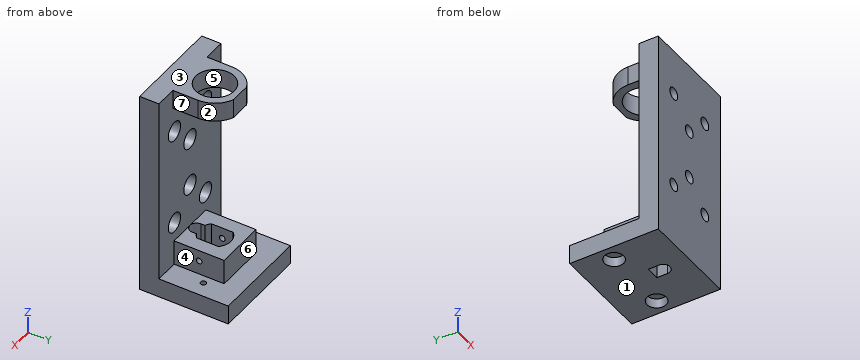
Autodesk Inventor part; units mm, degrees
ref_plane "Work Plane1" through (0, 0, 58.4) normal (0, 0, 1) x (1, 0, 0)
ref_plane "YZ Plane" through (0, 0, 0) normal (1, 0, 0) x (0, 1, 0)
ref_plane "XZ Plane" through (0, 0, 0) normal (0, 1, 0) x (-1, 0, 0)
sketch "Sketch1" plane through (0, 0, 0) normal (0, 0, 1) x (1, 0, 0)
  line L0 (-22.1831, 0) -> (-47.5831, 0)
  line L1 (0, 0) -> (50.8, 0)
  line L2 (50.8, 0) -> (50.8, 5)
  line L3 (50.8, 5) -> (50.8, 10)
  line L4 (50.8, 10) -> (50.8, 36)
  line L5 (50.8, 36) -> (50.8, 46)
  line L6 (50.8, 46) -> (0, 46)
  line L7 (0, 46) -> (0, 0)
  dimension "d0" = 25.4
  dimension "d1" = 50.8
  dimension "d2" = 5
  dimension "d3" = 5
  dimension "d4" = 26
  dimension "d5" = 10
extrude "Extrusion1" add sketch "Sketch1" along normal blind 10
sketch "Sketch2" plane through (0, 0, 10) normal (0, 0, 1) x (1, 0, 0)
  line L0 (50.8, 0) -> (50.8, 46)
  line L1 (50.8, 46) -> (0, 46)
  line L2 (0, 46) -> (0, 0)
  line L3 (0, 0) -> (50.8, 0)
  line L4 (0, 46) -> (0, 0)
  line L5 (0, 0) -> (50.8, 0)
  line L6 (50.8, 0) -> (50.8, 46)
  line L7 (50.8, 0) -> (50.8, 10)
  line L8 (50.8, 10) -> (0, 10)
  line L9 (0, 0) -> (0, 10)
  dimension "d8" = 10
extrude "Extrusion2" add sketch "Sketch2" along normal blind 87.5 contours L3 L2 L8 L0
sketch "Sketch3" plane through (0, 0, 10) normal (0, 0, 1) x (1, 0, 0)
  line L0 (0, 10) -> (50.8, 10)
  line L1 (50.8, 10) -> (50.8, 46)
  line L2 (50.8, 46) -> (0, 46)
  line L3 (0, 46) -> (0, 10)
  line L4 (12.4, 36) -> (38.4, 36)
  line L5 (38.4, 36) -> (38.4, 10)
  line L6 (38.4, 10) -> (12.4, 10)
  line L7 (12.4, 10) -> (12.4, 36)
  line L8 (17.4, 31) -> (33.4, 31)
  line L9 (33.4, 31) -> (33.4, 15)
  line L10 (33.4, 15) -> (17.4, 15)
  line L11 (17.4, 15) -> (17.4, 31)
  point P0 (0, 0)
  dimension "d1" = 50.8
  dimension "d12" = 38.4
  dimension "d13" = 10
  dimension "d14" = 5
  dimension "d15" = 5
  dimension "d16" = 16
  dimension "d17" = 16
  dimension "d18" = 5
  dimension "d19" = 5
  dimension "d24" = 26
  dimension "d26" = 26
extrude "Extrusion3" add sketch "Sketch3" along normal blind 13 contours L7 L4 L5 L0 | L8 L9 L10 L11
sketch "Sketch5" plane through (0, 0, 0) normal (0, 0, -1) x (-1, 0, 0)
  line L0 (-12.4, 36) -> (-38.4, 36)
  line L1 (-38.4, 36) -> (-38.4, 10)
  line L2 (-12.4, 10) -> (-12.4, 36)
  line L3 (0, 10) -> (-12.4, 10)
  line L4 (-50.8, 10) -> (-50.8, 46)
  line L5 (-50.8, 46) -> (0, 46)
  line L6 (0, 46) -> (0, 10)
  line L7 (0, 0) -> (-50.8, 0)
  line L8 (-50.8, 0) -> (-50.8, 10)
  line L9 (-50.8, 10) -> (0, 10)
  line L10 (0, 10) -> (0, 0)
  circle A0 centre (-42.8, 28) radius 1.42
  circle A1 centre (-8, 28) radius 1.42
  line L11 (-38.4, 10) -> (-50.8, 10)
  dimension "d29" = 2.84
  dimension "d30" = 2.84
  dimension "d31" = 8
  dimension "d32" = 8
  dimension "d33" = 8
  dimension "d34" = 8
extrude "Extrusion5" cut sketch "Sketch5" against normal blind 26 contours A0 | A1
sketch "Sketch9" plane through (0, 0, 0) normal (0, 0, -1) x (-1, 0, 0)
  circle A0 centre (-8, 28) radius 1.42
  circle A1 centre (-42.8, 28) radius 1.42
  line L0 (-50.8, 0) -> (-50.8, 46)
  line L1 (0, 0) -> (-50.8, 0)
  line L2 (0, 46) -> (0, 0)
  line L3 (-50.8, 46) -> (0, 46)
  circle A2 centre (-42.8, 28) radius 1.42
  circle A3 centre (-42.8, 28) radius 5
  circle A4 centre (-8, 28) radius 1.42
  circle A5 centre (-8, 28) radius 5
  dimension "d55" = 10
  dimension "d56" = 10
extrude "Extrusion9" cut sketch "Sketch9" against normal blind 5 contours A3 | A5
sketch "Sketch7" plane through (0, 0, 23) normal (0, 0, 1) x (1, 0, 0)
  line L0 (12.4, 36) -> (12.4, 10)
  line L1 (38.4, 10) -> (38.4, 36)
  line L2 (38.4, 36) -> (12.4, 36)
  circle A0 centre (25.4, 23) radius 8.25
  circle A1 centre (25.4, 23) radius 6
  line L3 (19.4, 28.6624) -> (19.4, 17.3376)
  line L4 (38.4, 10) -> (12.4, 10)
  line L5 (31.4, 28.6624) -> (31.4, 17.3376)
  point P0 (0, 0)
  dimension "d42" = 26
  dimension "d43" = 16.5
  dimension "d45" = 13
  dimension "d46" = 12
  dimension "d59" = 26
  dimension "d61" = 0
  dimension "d62" = 180
  dimension "d69" = 0
  dimension "d99" = 13
extrude "Extrusion7" cut sketch "Sketch7" against normal blind 14 contours L5 A1 L3 A0 | A0 L3 A1 L5 | A1
sketch "Sketch10" plane through (38.4, 10, 10) normal (1, 0, 0) x (0, 0, -1)
  line L0 (-13, 7.3376) -> (-13, 18.6624)
  line L1 (-13, 7.3376) -> (1, 7.3376)
  line L2 (1, 7.3376) -> (1, 18.6624)
  line L3 (-13, 18.6624) -> (1, 18.6624)
  circle A0 centre (-7.25, 13) radius 1.5
  point P0 (10, -10)
  dimension "d63" = 3
  dimension "d64" = 8.25
  dimension "d65" = 11.3247
  dimension "d66" = 5.6624
extrude "Extrusion10" cut sketch "Sketch10" against normal through all contours A0
sketch "Sketch11" plane through (0, 10, 97.5) normal (0, 1, 0) x (1, 0, 0)
  line L0 (38.4, 87.5) -> (38.4, 74.5)
  line L1 (38.4, 74.5) -> (12.4, 74.5)
  line L2 (12.4, 74.5) -> (12.4, 87.5)
  line L3 (0, 87.5) -> (12.4, 87.5)
  line L4 (0, 87.5) -> (0, 0)
  line L5 (50.8, 0) -> (0, 0)
  line L6 (50.8, 87.5) -> (50.8, 0)
  line L7 (38.4, 87.5) -> (50.8, 87.5)
  circle A0 centre (50.8, 77.2) radius 3.175
  circle A1 centre (38.1, 64.5) radius 3.175
  line L8 (38.4, 74.5) -> (12.4, 74.5)
  line L9 (38.4, 74.5) -> (25.4, 74.5)
  circle A2 centre (25.4, 77.2) radius 3.175
  circle A3 centre (12.7, 64.5) radius 3.175
  circle A4 centre (0, 77.2) radius 3.175
  circle A5 centre (-12.7, 64.5) radius 3.175
  circle A6 centre (-25.4, 77.2) radius 3.175
  circle A7 centre (-38.1, 64.5) radius 3.175
  circle A8 centre (50.8, 51.8) radius 3.175
  circle A9 centre (38.1, 39.1) radius 3.175
  circle A10 centre (25.4, 51.8) radius 3.175
  circle A11 centre (12.7, 39.1) radius 3.175
  circle A12 centre (0, 51.8) radius 3.175
  circle A13 centre (-12.7, 39.1) radius 3.175
  circle A14 centre (-25.4, 51.8) radius 3.175
  circle A15 centre (-38.1, 39.1) radius 3.175
  circle A16 centre (50.8, 26.4) radius 3.175
  circle A17 centre (38.1, 13.7) radius 3.175
  circle A18 centre (25.4, 26.4) radius 3.175
  circle A19 centre (12.7, 13.7) radius 3.175
  circle A20 centre (0, 26.4) radius 3.175
  circle A21 centre (-12.7, 13.7) radius 3.175
  circle A22 centre (-25.4, 26.4) radius 3.175
  circle A23 centre (-38.1, 13.7) radius 3.175
  circle A24 centre (50.8, 1) radius 3.175
  circle A25 centre (38.1, -11.7) radius 3.175
  circle A26 centre (25.4, 1) radius 3.175
  circle A27 centre (12.7, -11.7) radius 3.175
  circle A28 centre (0, 1) radius 3.175
  circle A29 centre (-12.7, -11.7) radius 3.175
  circle A30 centre (-25.4, 1) radius 3.175
  circle A31 centre (-38.1, -11.7) radius 3.175
  point P0 (0, 97.5)
  dimension "d70" = 26
  dimension "d71" = 6.35
  dimension "d72" = 6.35
  dimension "d73" = 13
  dimension "d75" = 12.7
  dimension "d76" = 12.7
  dimension "d77" = 10.3
  dimension "d78" = 13
  dimension "d82" = 25.4
  dimension "d85" = 25.4
  dimension "d88" = 12.7
extrude "Extrusion11" cut sketch "Sketch11" against normal blind 10 contours A1 | A3 | A10
sketch "Sketch12" plane through (0, 10, 97.5) normal (0, 1, 0) x (1, 0, 0)
  circle A0 centre (38.1, 64.5) radius 3.175
  circle A1 centre (25.4, 51.8) radius 3.175
  circle A2 centre (12.7, 64.5) radius 3.175
  line L0 (38.4, 87.5) -> (38.4, 74.5)
  line L1 (38.4, 74.5) -> (12.4, 74.5)
  line L2 (12.4, 74.5) -> (12.4, 87.5)
  line L3 (0, 87.5) -> (12.4, 87.5)
  line L4 (0, 87.5) -> (0, 0)
  line L5 (50.8, 0) -> (0, 0)
  line L6 (50.8, 87.5) -> (50.8, 0)
  line L7 (38.4, 87.5) -> (50.8, 87.5)
  circle A3 centre (12.7, 64.5) radius 5
  circle A4 centre (25.4, 51.8) radius 5
  circle A5 centre (38.1, 64.5) radius 3.175
  circle A6 centre (38.1, 64.5) radius 5
  point P0 (0, 97.5)
  dimension "d91" = 10
  dimension "d92" = 10
  dimension "d93" = 10
extrude "Extrusion12" cut sketch "Sketch12" against normal blind 5 contours A0 | A1 | A2 | A3 | A4 | A6
sketch "Sketch14" plane through (0, 0, 97.5) normal (0, 0, 1) x (1, 0, 0)
  line L0 (7.7, 5) -> (17.7, 5)
  line L1 (50.8, 10) -> (0, 10)
  line L2 (0, 10) -> (0, 0)
  line L3 (0, 0) -> (50.8, 0)
  line L4 (50.8, 0) -> (50.8, 10)
  circle A0 centre (25.4, 23) radius 10
  circle A1 centre (25.4, 23) radius 14
  line L5 (0, 46) -> (0, 0)
  line L6 (0, 0) -> (50.8, 0)
  line L7 (50.8, 0) -> (50.8, 10)
  line L8 (50.8, 10) -> (0, 10)
  line L9 (0, 10) -> (0, 0)
  circle A2 centre (8, 28) radius 1.42
  circle A3 centre (42.8, 28) radius 1.42
  line L10 (38.4, 36) -> (38.4, 10)
  line L11 (38.4, 10) -> (50.8, 10)
  line L12 (50.8, 10) -> (50.8, 46)
  line L13 (50.8, 46) -> (0, 46)
  line L14 (0, 46) -> (0, 10)
  line L15 (0, 10) -> (12.4, 10)
  line L16 (12.4, 10) -> (12.4, 36)
  line L17 (12.4, 36) -> (38.4, 36)
  circle A4 centre (8, 28) radius 1.42
  circle A5 centre (8, 28) radius 3
  circle A6 centre (42.8, 28) radius 1.42
  circle A7 centre (42.8, 28) radius 3
  line L18 (11.4, 23) -> (11.4, 10)
  line L19 (39.4, 23) -> (39.4, 10)
  line L20 (33.1, 10) -> (43.1, 10)
  circle A8 centre (25.4, 23) radius 9
  line L21 (19.4, 17.3376) -> (19.4, 28.6624)
  arc A9 (19.4, 17.3376) -> (31.4, 17.3376) centre (25.4, 23) ccw
  line L22 (31.4, 28.6624) -> (31.4, 17.3376)
  arc A10 (31.4, 28.6624) -> (19.4, 28.6624) centre (25.4, 23) ccw
  line L23 (12.4, 36) -> (12.4, 10)
  line L24 (39.4, 10) -> (12.4, 10)
  line L25 (12.4, 10) -> (12.4, 36)
  line L26 (12.4, 36) -> (39.4, 36)
  line L27 (39.4, 36) -> (39.4, 10)
  point P0 (12.4, 10)
  point P1 (38.4, 28.1962)
  point P2 (30.5962, 36)
  point P3 (20.2038, 36)
  point P4 (12.4, 28.1962)
  point P5 (38.4, 17.8038)
  point P6 (12.4, 17.8038)
  dimension "d100" = 20
  dimension "d101" = 28
  dimension "d102" = 6
  dimension "d103" = 6
  dimension "d106" = 18
  dimension "d107" = 0
  dimension "d117" = 0
extrude "Extrusion14" add sketch "Sketch14" along normal blind 10 contours L4 L3 L2 L1 A1 | L1 L10 A1 L19 | L1 A1 L10 | A1 L10 | A1 L1 L16 L17 L10 | L18 A1 L16 L1 | A1 L1 | L16 A1 L1 | A1 L16
ref_plane "Work Plane1" through (0, 0, 58.4) normal (0, 0, 1) x (1, 0, 0)
mirror "Mirror1" about plane through (0, 0, 58.4) normal (0, 0, 1) of "Extrusion12", "Extrusion11"
sketch "Sketch15" plane through (0, 0, 23) normal (0, 0, 1) x (1, 0, 0)
  arc A0 (31.4, 28.6624) -> (19.4, 28.6624) centre (25.4, 23) ccw
  line L0 (19.4, 17.3376) -> (19.4, 28.6624)
  arc A1 (19.4, 17.3376) -> (31.4, 17.3376) centre (25.4, 23) ccw
  line L1 (31.4, 28.6624) -> (31.4, 17.3376)
  line L2 (19.4, 17.3376) -> (19.4, 28.6624)
  arc A2 (31.4, 28.6624) -> (19.4, 28.6624) centre (25.4, 23) ccw
  line L3 (31.4, 28.6624) -> (31.4, 17.3376)
  arc A3 (19.4, 17.3376) -> (31.4, 17.3376) centre (25.4, 23) ccw
  line L4 (12.4, 36) -> (12.4, 10)
  line L5 (38.4, 10) -> (12.4, 10)
  line L6 (38.4, 10) -> (38.4, 36)
  line L7 (38.4, 36) -> (12.4, 36)
  circle A4 centre (25.4, 13.5) radius 3.5
  line L8 (28.9, 26.8597) -> (21.9, 26.8597)
  line L9 (21.9, 11.25) -> (28.9, 11.25)
  line L10 (28.9, 11.25) -> (28.9, 19)
  line L11 (28.9, 19) -> (21.9, 19)
  line L12 (21.9, 19) -> (21.9, 11.25)
  point P0 (0, 0)
  point P1 (21.9, 13.5)
  point P2 (28.9, 13.5)
  dimension "d109" = 7
  dimension "d110" = 0
  dimension "d111" = 8.25
  dimension "d113" = 3.5
  dimension "d116" = 5.5
extrude "Extrusion15" cut sketch "Sketch15" against normal through all contours L10 A4 A1 | A1 A4 L12 L11 L10 | A1 A4 L12 | A4 L9 A1 | A1 A4 | A4 L9
equation "\"d8\" = d2 + d3"
equation "\"d12\" = 0.5 * d26 + 0.5 * d1"
equation "\"d15\" = d14"
equation "\"d17\" = d16"
equation "\"d18\" = d14"
equation "\"d19\" = d14"
equation "\"d30\" = d29"
equation "\"d32\" = d31"
equation "\"d33\" = d31"
equation "\"d34\" = d31"
equation "\"d35\" = d26"
equation "\"d56\" = d55"
equation "\"d45\" = 0.5 * d42"
equation "\"d66\" = 0.5 * d65"
equation "\"d71\" = 0.25 * d0"
equation "\"d72\" = d71"
equation "\"d73\" = 0.5 * d70"
equation "\"d75\" = 0.5 * d0"
equation "\"d76\" = 0.5 * d0"
equation "\"d82\" = d0"
equation "\"d85\" = d0"
equation "\"d88\" = 0.5 * d0"
equation "\"d92\" = d91"
equation "\"d93\" = d91"
equation "\"d113\" = 0.5 * d109"
properties part number "Actuator Stage Actuator Mount V0.2"
Geometry check sheet. Reference: the model listing, model coordinates, mm. Face numbers are marked on the shaded views. A direction names the side the tool comes from. Coordinates: 2 decimals unless noted, no trailing zeros. Order: outer loops, then holes, each group sorted by start corner. A loop starts at its lowest first (then second) coordinate and runs counter-clockwise, first axis right, second up. Notation, with made-up numbers: M 58.25,-14.75 L 109.25,-14.75 A13 ccw 109.25,9.25 Z; hole C 67,73 d5. An arc over 180 degrees is marked long. Use CSV: the item, a comma, the result in double quotes.
Item 1: Tool access check on the marked faces 5, 6 and 7. Record the directions out of +Z, -Z, +X, -X, +Y, -Y that give a thin tool (end or side, any length) a straight path to the whole face; none if there is none.
Returned:
face 5,"+Z"
face 6,"+Z, +X, -X, +Y"
face 7,"+Z, +X, +Y"
Item 2: Cross-section at C-C on y = 38.5. Record the cut outline in (x, z).
Returned:
outline,"M 0,0 L 50.8,0 L 50.8,10 L 0,10 Z"
Item 3: Cross-section at B-B on z = 33. Record the cut outline in (x, y) (3 decimals).
Returned:
outline,"M 0,0 L 9.525,0 L 9.525,5 L 7.7,5 L 7.7,10 L 0,10 Z; M 15.875,0 L 34.925,0 L 34.925,5 L 33.1,5 L 33.1,10 L 17.7,10 L 17.7,5 L 15.875,5 Z; M 41.275,0 L 50.8,0 L 50.8,10 L 43.1,10 L 43.1,5 L 41.275,5 Z"
Item 4: Gauge pin test, flat ends, axial feed: pin 1 Ø5 at (x, y) = (42, 29) entering from -Z; pin 2 Ø14.5 at (y, z) = (17.5, 19) entering from +X; pin 3 Ø7.5 at (x, z) = (12.7, 33) entering from +Y. Record the tip position at first contact, or that the pin passes through.
Returned:
pin 1,"stops at z = 5"
pin 2,"stops at x = 38.4"
pin 3,"stops at y = 5"
Item 5: Thickness scan on line 1 along X through (y, z) = (6, 33); line 2 along Y through (x, z) = (8, 7.25); line 3 along Z through (x, y) = (17, 17). Record the ranges inside material, lowest first.
Returned:
line 1,"x = 0 to 7.7, 17.7 to 33.1, 43.1 to 50.8"
line 2,"y = 0 to 26.58, 29.42 to 46"
line 3,"z = 0 to 23, 97.5 to 107.5"
Item 6: Cross-section at A-A on z = 71.1. Record the cut outline in (x, y) (3 decimals), then the cut area to 3 significant figures.
Returned:
outline,"M 0,0 L 22.225,0 L 22.225,5 L 20.4,5 L 20.4,10 L 0,10 Z; M 28.575,0 L 50.8,0 L 50.8,10 L 30.4,10 L 30.4,5 L 28.575,5 Z"
area,"426 mm2"
Item 7: Mould release check, pull along Z, two halves, no side actions. Record for the marked faces 1, 2, 3 and 4: pulls with the +Z half, pulls with the -Z half, needs draft (parallel to the pull), parting line crosses it, or undercut.
Returned:
face 1,"pulls with the -Z half"
face 2,"needs draft"
face 3,"pulls with the +Z half"
face 4,"undercut"
